from build123d import *

# Parameters (mm, degrees)
SKETCH1_R               = 10.5
BOSS_EXTRUDE2_DEPTH     = 3
SKETCH2_R               = 6
BOSS_EXTRUDE3_DEPTH     = 10
SKETCH3_R               = 4.5
CUT_EXTRUDE1_DEPTH      = 4
SKETCH4_R               = 8.75
BOSS_EXTRUDE4_DEPTH     = 8
CHAMFER1_SIZE           = 3
SKETCH5_R               = 7.15
CUT_EXTRUDE3_DEPTH      = 8
SKETCH6_R               = 1.5
CUT_EXTRUDE4_DEPTH      = 9
CUT_EXTRUDE5_REACH      = 27.72
CUT_EXTRUDE5_END_RADIUS = 8.75
SKETCH7_R               = 2


with BuildPart() as part:
    # Sketch1 → Boss-Extrude2 (new body)
    with BuildSketch(Plane.XY):
        Circle(SKETCH1_R)
    extrude(amount=BOSS_EXTRUDE2_DEPTH)

    # Sketch2 → Boss-Extrude3 (add)
    with BuildSketch(Plane.XY.offset(3)):
        Circle(SKETCH2_R)
    extrude(amount=BOSS_EXTRUDE3_DEPTH)

    # Sketch3 → Cut-Extrude1 (cut)
    with BuildSketch(Plane.XY.offset(13)):
        Circle(SKETCH3_R)
    extrude(amount=-CUT_EXTRUDE1_DEPTH, mode=Mode.SUBTRACT)

    # Sketch4 → Boss-Extrude4 (add)
    with BuildSketch(Plane.XY.offset(13)):
        Circle(SKETCH4_R)
    extrude(amount=BOSS_EXTRUDE4_DEPTH)

    # Chamfer1
    # the kernel refuses this chamfer: 3 mm, written as the material it adds along each edge
    with BuildSketch(Plane(origin=(0, 0, 13), x_dir=(1, 0, 0), z_dir=(0, -1, 0))) as chamfer1_piece_1_section:
        Polygon((6 + CHAMFER1_SIZE, 0), (6, -CHAMFER1_SIZE), (6, 0), align=None)
    chamfer1_piece_1 = revolve(axis=Axis((0, 0, 13), (0, 0, 1)), mode=Mode.PRIVATE)
    chamfer1_piece_1 = chamfer1_piece_1 & Plane(origin=(0, 0, 11.374833607), x_dir=(1, 0, 0), z_dir=(0, 0, -1)) * Cylinder(8.75, 36, mode=Mode.PRIVATE)
    add(chamfer1_piece_1)

    # Sketch5 → Cut-Extrude3 (cut)
    with BuildSketch(Plane.XY.offset(21)):
        Circle(SKETCH5_R)
    extrude(amount=-CUT_EXTRUDE3_DEPTH, mode=Mode.SUBTRACT)

    # Sketch6 → Cut-Extrude4 (cut)
    with BuildSketch(Plane.XY.offset(9)):
        Circle(SKETCH6_R)
    extrude(amount=-CUT_EXTRUDE4_DEPTH, mode=Mode.SUBTRACT)

    # Cut-Extrude5: up to this cylinder (the profile starts inside it)
    cut_extrude5_end = Plane(origin=(0, 0, 16.5), z_dir=(0, 0, -1)) * Cylinder(CUT_EXTRUDE5_END_RADIUS, 73.94, mode=Mode.PRIVATE)
    # Sketch7 → Cut-Extrude5 (cut, up to the surface)
    with BuildSketch(Plane(origin=(0, 0, 0), x_dir=(0, 0, -1), z_dir=(1, 0, 0)), mode=Mode.PRIVATE) as cut_extrude5_sk1:
        with Locations((-16.5, 0)):
            Circle(SKETCH7_R)
    cut_extrude5_tool1 = extrude(cut_extrude5_sk1.sketch, amount=-CUT_EXTRUDE5_REACH, mode=Mode.PRIVATE) & cut_extrude5_end
    add(cut_extrude5_tool1.solids().sort_by_distance((0, 0, 16.5))[0], mode=Mode.SUBTRACT)


solid = part.part
Can you work these out from the model? Positions are in its coordinate system, mm. A direction names the side the tool comes from. Round coordinates to 2 decimals unless told otherwise and drop trailing zeros. Loops run counter-clockwise (first coordinate to the right, second up) from the corner with the lowest first, then second, coordinate; pieces in that order, holes last. Notation, with made-up numbers: (71.5, -40) - (120.5, -40) arc R21 ccw to (120.5, -24) - close; hole circle Ø8 at (75, -35.75). An arc over 180 degrees is marked (long way). Write item = value, one per line. Start each with the question number.
(1) If we section it at A-A (y = 0): Please give me the cut outline in (x, z), and give its area (3 significant figures).
(2) If we section it at B-B (x = 0): Please give me the cut outline in (y, z), and give its area (3 significant figures).
(3) If we section it at D-D (z = 10.5): Please give me the cut outline in (x, y).
(4) For P1, Ø4, axis at y = -4.5, z = 13.5, coming from the +X side; P2, Ø5, axis at y = 0, z = 16.5, coming from the +X side; P3, Ø5, axis at x = 0, y = 0, coming from the +Z side; P4, Ø8, axis at x = 1.5, y = 4.5, coming from the -Z side, each with a flat end and sliding along its axis, tell me the tip position at first contact or that it passes through.
(5) If we mould it in two halves opening along Z, with no side actions, what happens to faces 1 (the face through (-7.8, -1.2, 18.1)), 2 (the face through (0, -2, 9)), 3 (the face through (2, 0, 0)), 4 (the face through (-6, 0, 6))? For each: released by +Z, released by -Z, zero draft, split by the parting line, or undercut.
(6) If we section it at C-C (z = 3.75): Please give me the cut outline in (x, y), and give its area (3 significant figures).
(7) For faces 5 (the face through (5, -5, 3)), 6 (the face through (-1.5, 0.07, 4.56)), 7 (the face through (-0.59, 4.46, 11.03)), which set-ups out of +Z, -Z, +X, -X, +Y, -Y let a thin tool reach every point of the face, with its end or its side?
(8) If I drill on probe 1 along Y at (x, z) = (0, 3.25); probe 2 along Y at (x, z) = (0, 16); probe 3 along Z at (x, y) = (-8.25, 0.5), over which ranges is the centre line in solid material (lowest first)? Write a range as [from, to].
Ans:
q1.outline = (-10.5, 0) - (-1.5, 0) - (-1.5, 9) - (-4.5, 9) - (-4.5, 13) - (-7.15, 13) - (-7.15, 14.5) - (-8.75, 14.5) - (-8.75, 12.75) - (-6, 10) - (-6, 3) - (-10.5, 3) - close; (-8.75, 18.5) - (-7.15, 18.5) - (-7.15, 21) - (-8.75, 21) - close; (1.5, 0) - (10.5, 0) - (10.5, 3) - (6, 3) - (6, 10) - (8.75, 12.75) - (8.75, 21) - (7.15, 21) - (7.15, 13) - (4.5, 13) - (4.5, 9) - (1.5, 9) - close
q1.area = 148 mm²
q2.outline = (-10.5, 0) - (-1.5, 0) - (-1.5, 9) - (-4.5, 9) - (-4.5, 13) - (-7.15, 13) - (-7.15, 21) - (-8.75, 21) - (-8.75, 12.75) - (-6, 10) - (-6, 3) - (-10.5, 3) - close; (1.5, 0) - (10.5, 0) - (10.5, 3) - (6, 3) - (6, 10) - (8.75, 12.75) - (8.75, 21) - (7.15, 21) - (7.15, 13) - (4.5, 13) - (4.5, 9) - (1.5, 9) - close
q2.area = 155 mm²
q3.outline = circle Ø13 at (0, 0); hole circle Ø9 at (0, 0)
q4.P1 = 8.39
q4.P2 = 8.75
q4.P3 = 9
q4.P4 = 0
q5.face_1 = undercut
q5.face_2 = released by +Z
q5.face_3 = released by -Z
q5.face_4 = undercut
q6.outline = circle Ø12 at (0, 0); hole circle Ø3 at (0, 0)
q6.area = 106 mm²
q7.face_5 = none
q7.face_6 = +Z, -Z
q7.face_7 = +Z
q8.probe_1 = [-6, -1.5], [1.5, 6]
q8.probe_2 = [-8.75, -7.15], [7.15, 8.75]
q8.probe_3 = [0, 3], [12.27, 14.56], [18.44, 21]
